Here's how the part is built. I have some questions about the finished solid (model axes, mm). Face numbers are marked on the shaded views. A direction names the side the tool comes from. Give positions to 0.01 mm unless a question says otherwise; leave off trailing zeros. Loops run counter-clockwise (first coordinate to the right, second up) from the corner with the lowest first, then second, coordinate; pieces in that order, holes last. Notation, with made-up numbers: (59.25, 19.25) -> (93.25, 19.25) arc R25 cw to (93.25, 49.25) -> close; hole circle Ø2 at (88, 28). An arc over 180 degrees is marked (long way). Answer in a Markdown table with one row per item. Add a question column.
Item 1: For P1, Ø5, axis at x = -2, z = -10.5, coming from the +Y side; P2, Ø1.3, axis at x = -1, z = -27.5, coming from the +Y side; P3, Ø1.3, axis at x = 0, z = -27, coming from the -Y side, each with a flat end and sliding along its axis, tell me the tip position at first contact or that it passes through.
Item 2: If I drill on line 1 (X direction, y = -1.7, z = -10); line 2 (Z direction, x = 2.75, y = -1.65); line 3 (X direction, y = -0.05, z = 18.5), over which ranges is the centre line in solid material (lowest first)?
Item 3: If we section it at B-B (x = 0): Write out the boundary of the cut face in (y, z), then the cut area to 3 significant figures.
Item 4: Which directions (+Z, -Z, +X, -X, +Y, -Y) give clear straight access to the entire face, cutting with the end or side of a thin tool? Please do the marked faces 1 and 2.
Item 5: If we section it at D-D (z = 16): Write out the boundary of the cut face in (x, y), then the cut area to 3 significant figures.
Item 6: If we section it at A-A (y = 1.3): Write out the boundary of the cut face in (x, z).
Item 7: If we section it at C-C (z = -4): Write out the boundary of the cut face in (x, y), then the cut area to 3 significant figures.
Autodesk Inventor part; units mm, degrees
ref_plane "YZ Plane" through (0, 0, 0) normal (1, 0, 0) x (0, 1, 0)
ref_plane "XZ Plane" through (0, 0, 0) normal (0, 1, 0) x (-1, 0, 0)
ref_plane "XY Plane" through (0, 0, 0) normal (0, 0, 1) x (1, 0, 0)
sketch "Sketch1" plane through (0, 0, 0) normal (0, 0, 1) x (1, 0, 0)
  line L0 (-10, 2.25) -> (10, 2.25)
  line L1 (10, 2.25) -> (10, -2.25)
  line L2 (10, -2.25) -> (-10, -2.25)
  line L3 (-10, -2.25) -> (-10, 2.25)
  line L4 (-10, 2.25) -> (10, -2.25) construction
  line L5 (10, 2.25) -> (-10, -2.25) construction
  line L6 (-2.25, 3.75) -> (2.25, 3.75)
  line L7 (2.25, 3.75) -> (2.25, 0.75)
  line L8 (2.25, 0.75) -> (-2.25, 0.75)
  line L9 (-2.25, 0.75) -> (-2.25, 3.75)
  line L10 (-2.25, 3.75) -> (2.25, 0.75) construction
  line L11 (2.25, 3.75) -> (-2.25, 0.75) construction
  line L12 (-2.25, -0.6661) -> (2.25, -0.6661)
  line L13 (2.25, -0.6661) -> (2.25, -3.8339)
  line L14 (2.25, -3.8339) -> (-2.25, -3.8339)
  line L15 (-2.25, -3.8339) -> (-2.25, -0.6661)
  line L16 (-2.25, -0.6661) -> (2.25, -3.8339) construction
  line L17 (2.25, -0.6661) -> (-2.25, -3.8339) construction
  point P0 (0, 0)
  point P1 (0, 2.25)
  point P2 (0, -2.25)
  point P3 (2.25, 2.25)
  point P4 (-2.25, 2.25)
  point P5 (-2.25, -2.25)
  point P6 (2.25, -2.25)
  dimension "d0" = 20
  dimension "d1" = 4.5
  dimension "d2" = 4.5
  dimension "d3" = 3
extrude "Extrusion1" add sketch "Sketch1" along normal mid plane 60 contours L0 L9 L8 L7 L1 L2 L13 L12 L15 L3
sketch "Sketch2" plane through (2.25, 2.25, 30) normal (0, 1, 0) x (1, 0, 0)
  line L0 (-5.35, 13) -> (0.85, 13)
  line L1 (0.85, 13) -> (0.85, 8)
  line L2 (0.85, 8) -> (-5.35, 8)
  line L3 (-5.35, 8) -> (-5.35, 13)
  line L4 (-5.35, 13) -> (0.85, 8) construction
  line L5 (0.85, 13) -> (-5.35, 8) construction
  line L6 (0, 0) -> (-4.5, 0)
  circle A0 centre (-2.25, 8) radius 3.1
  circle A1 centre (-2.25, 13) radius 3.1
  line L7 (7.75, 0) -> (7.75, 60)
  line L8 (7.75, 30) -> (-12.25, 30)
  line L9 (-12.25, 60) -> (-12.25, 0)
  line L10 (0.85, 47) -> (0.85, 52)
  line L11 (-5.35, 52) -> (-5.35, 47)
  circle A2 centre (-2.25, 52) radius 3.1
  circle A3 centre (-2.25, 47) radius 3.1
  point P0 (-2.25, 30)
  point P1 (-2.25, 10.5)
  point P2 (-2.25, 49.5)
  dimension "d6" = 6.2
  dimension "d7" = 5
  dimension "d8" = 8
extrude "Extrusion2" cut sketch "Sketch2" against normal blind 60
properties part number "Spacer Laser"
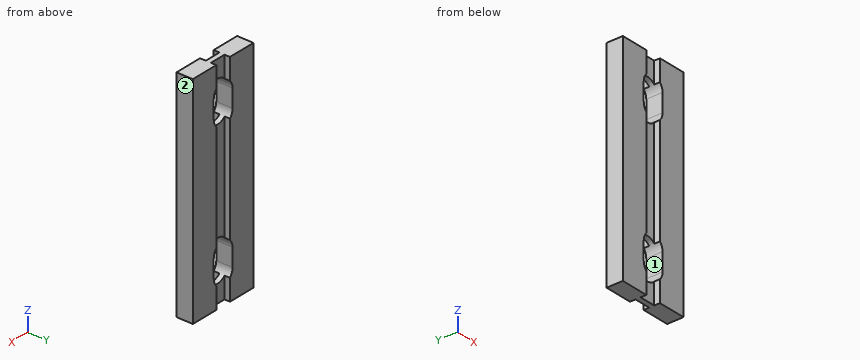
Recorded:
| question | item | result |
|---|---|---|
| 1 | P1 | stops at y = 2.25 |
| 1 | P2 | stops at y = 0.75 |
| 1 | P3 | stops at y = -0.67 |
| 2 | line 1 | x = -10 to -2.25, 2.25 to 10 |
| 2 | line 2 | z = -30 to -23.43, -15.57 to 15.57, 23.43 to 30 |
| 2 | line 3 | x = -10 to -3.1, 3.1 to 10 |
| 3 | outline | (-0.67, -30) -> (0.75, -30) -> (0.75, -25.1) -> (-0.67, -25.1) -> close; (-0.67, -13.9) -> (0.75, -13.9) -> (0.75, 13.9) -> (-0.67, 13.9) -> close; (-0.67, 25.1) -> (0.75, 25.1) -> (0.75, 30) -> (-0.67, 30) -> close |
| 3 | area | 53.2 mm^2 |
| 4 | face 1 | +Y, -Y |
| 4 | face 2 | +Z, -Z, +X, +Y, -Y |
| 5 | outline | (-10, -2.25) -> (-2.93, -2.25) -> (-2.93, 2.25) -> (-10, 2.25) -> close; (2.93, -2.25) -> (10, -2.25) -> (10, 2.25) -> (2.93, 2.25) -> close |
| 5 | area | 63.6 mm^2 |
| 6 | outline | (-10, -30) -> (-2.25, -30) -> (-2.25, -24.13) arc R3.1 cw to (-3.1, -22) -> (-3.1, -17) arc R3.1 cw to (-2.25, -14.87) -> (-2.25, 14.87) arc R3.1 cw to (-3.1, 17) -> (-3.1, 22) arc R3.1 cw to (-2.25, 24.13) -> (-2.25, 30) -> (-10, 30) -> close; (2.25, -30) -> (10, -30) -> (10, 30) -> (2.25, 30) -> (2.25, 24.13) arc R3.1 cw to (3.1, 22) -> (3.1, 17) arc R3.1 cw to (2.25, 14.87) -> (2.25, -14.87) arc R3.1 cw to (3.1, -17) -> (3.1, -22) arc R3.1 cw to (2.25, -24.13) -> close |
| 7 | outline | (-10, -2.25) -> (-2.25, -2.25) -> (-2.25, -0.67) -> (2.25, -0.67) -> (2.25, -2.25) -> (10, -2.25) -> (10, 2.25) -> (2.25, 2.25) -> (2.25, 0.75) -> (-2.25, 0.75) -> (-2.25, 2.25) -> (-10, 2.25) -> close |
| 7 | area | 76.1 mm^2 |
